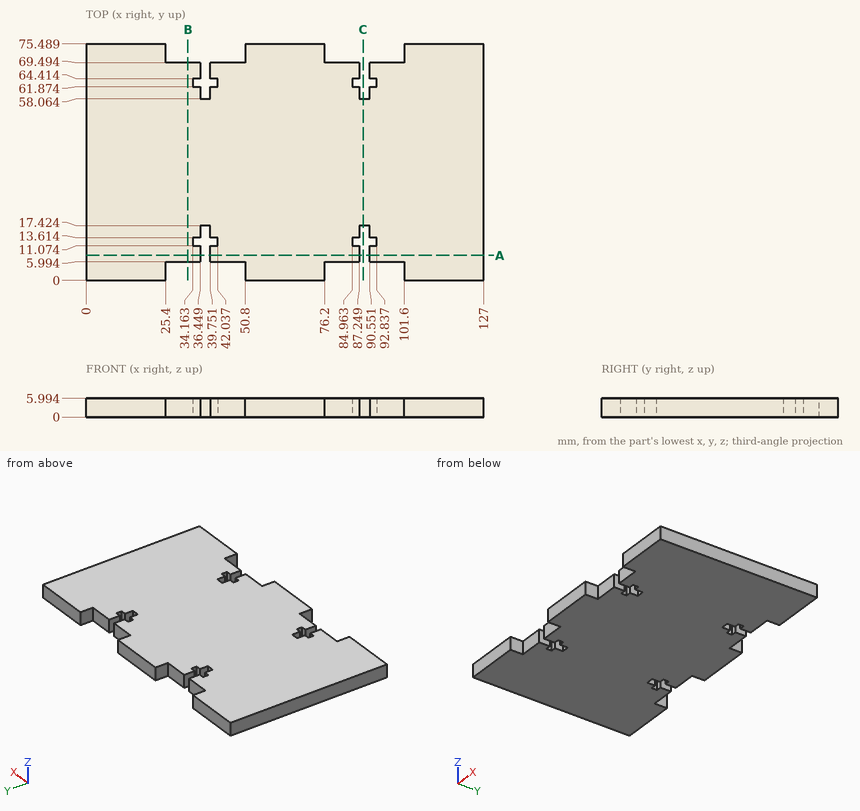
Geometry: see drawing. Coordinates: mm, zero at the bounding-box minimum. Round coordinates to 2 decimals unless told otherwise and drop trailing zeros. Loops run counter-clockwise (first coordinate to the right, second up) from the corner with the lowest first, then second, coordinate; pieces in that order, holes last. Notation, with made-up numbers: (13.25, -36.5) - (57.25, -36.5) arc R15 cw to (57.25, -8.5) - close; hole circle Ø11 at (41.25, 24.25). An arc over 180 degrees is marked (long way). Write item = value, one per line. Start each with the question number.
(1) Section query A-A, the plane y = 8. Output: boundary loops of the cut face in (x, z) (1 decimal).
(2) Section query C-C, the plane x = 88.5. Output: boundary loops of the cut face in (y, z) (1 decimal), plus the area to 3 significant figures.
(3) Ray query, line 1 along X through (y, z) = (64.5, 5.6); line 2 along Y through (x, z) = (85, 3.65) (1 decimal); line 3 along Y through (x, z) = (94, 3.9) (1 decimal). Return the intervals inside material, ascending. Write a range as from..to.
(4) Section query B-B, the plane x = 32.5. Output: boundary loops of the cut face in (y, z) (1 decimal), plus the area to 3 significant figures.
(5) Pin query (flat end, axial travel): pin 1 (2.5 mm diameter, centred on x = 40.5, z = 3, fed in from -Y); pin 2 (2.5 mm diameter, centred on x = 35, z = 1.5, fed in from +Y); pin 3 (12 mm diameter, centred on x = 107.5, y = 10, fed in from -Z). Return the tip coordinate at first contact, or that it passes through.
Conclusion:
q1.outline = (0, 0) - (36.4, 0) - (36.4, 6) - (0, 6) - close; (39.8, 0) - (87.2, 0) - (87.2, 6) - (39.8, 6) - close; (90.6, 0) - (127, 0) - (127, 6) - (90.6, 6) - close
q2.outline = (17.4, 0) - (58.1, 0) - (58.1, 6) - (17.4, 6) - close
q2.area = 244 mm2
q3.line_1 = 0..36.45, 39.75..87.25, 90.55..127
q3.line_2 = 6..11.1, 13.6..61.9, 64.4..69.5
q3.line_3 = 6..69.5
q4.outline = (6, 0) - (69.5, 0) - (69.5, 6) - (6, 6) - close
q4.area = 381 mm2
q5.pin_1 = 5.99
q5.pin_2 = 69.49
q5.pin_3 = 0
